Build history of the part. All positions in model axes, mm. Round coordinates to 2 decimals unless told otherwise and drop trailing zeros. Order: outer loops, then holes, each group sorted by start corner. A loop starts at its lowest first (then second) coordinate and runs counter-clockwise, first axis right, second up. Notation, with made-up numbers: (-15.5, 61.5) - (-9.5, 61.5) arc R24 ccw to (-9.5, 98.5) - close; hole circle Ø5 at (-25.75, -29.5). An arc over 180 degrees is marked (long way). Write each question's results on one line, items separated by ' | '. Start each with the question number.
```python
from build123d import *

# Parameters (mm, degrees)
SKETCH1_W           = 10.16
SKETCH1_H           = 3.175
BOSS_EXTRUDE1_DEPTH = 3.175


with BuildPart() as part:
    # Sketch1 → Boss-Extrude1 (new body)
    with BuildSketch(Plane(origin=(0, 0, 0), x_dir=(1, 0, 0), z_dir=(0, 1, 0))):
        with Locations((22.86, -42.8625)):
            Rectangle(SKETCH1_W, SKETCH1_H)
        Polygon((27.94, -41.275), (38.1, -41.275), (48.26, -41.275), (58.42, -41.275), (68.58, -41.275), (76.2, -41.275), (76.2, 41.275), (68.58, 41.275), (58.42, 41.275), (48.26, 41.275), (38.1, 41.275), (27.94, 41.275), (17.78, 41.275), (-76.2, 41.275), (-76.2, -41.275), (17.78, -41.275), align=None)
        with Locations((43.18, -42.8625)):
            Rectangle(SKETCH1_W, SKETCH1_H)
        with Locations((22.86, 42.8625)):
            Rectangle(SKETCH1_W, SKETCH1_H)
        with Locations((63.5, -42.8625)):
            Rectangle(SKETCH1_W, SKETCH1_H)
        with Locations((63.5, 42.8625)):
            Rectangle(SKETCH1_W, SKETCH1_H)
        with Locations((43.18, 42.8625)):
            Rectangle(SKETCH1_W, SKETCH1_H)
    extrude(amount=BOSS_EXTRUDE1_DEPTH)


solid = part.part
```
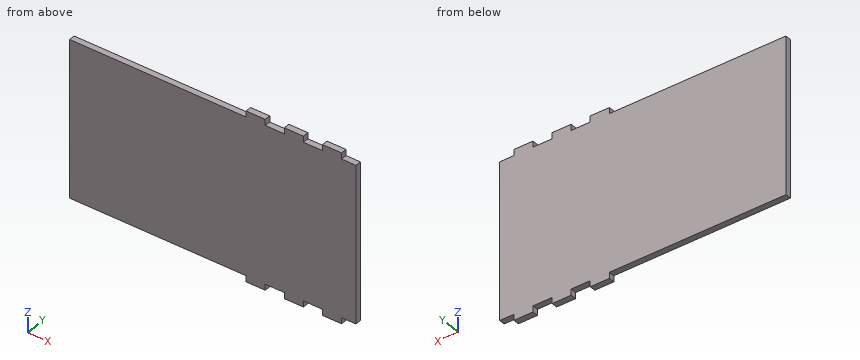
1. Wall check: line 1 (Z direction, x = 6, y = 0.95) (3 decimals). Give the ranges that are in metal, low to high. Write a range as from..to.
2. Cut at A-A (y = 1.45). List the corners of the cut face in (x, z) (3 decimals), plus the area to 3 significant figures.
3. Flat gauge pins, fed straight in: pin 1 Ø1 at (y, z) = (1.5, -42.5) entering from -X; pin 2 Ø1.6 at (x, y) = (-34.5, 2) entering from +Z (3 decimals); pin 3 Ø1.6 at (x, y) = (35, 2) entering from -Z (3 decimals). Where does each tip first touch, or does it go through?
4. Cut at B-B (x = 14). List the corners of the cut face in (y, z) (3 decimals).
A:
1) line 1: z = -41.275..41.275
2) outline: (-76.2, -41.275) - (17.78, -41.275) - (17.78, -44.45) - (27.94, -44.45) - (27.94, -41.275) - (38.1, -41.275) - (38.1, -44.45) - (48.26, -44.45) - (48.26, -41.275) - (58.42, -41.275) - (58.42, -44.45) - (68.58, -44.45) - (68.58, -41.275) - (76.2, -41.275) - (76.2, 41.275) - (68.58, 41.275) - (68.58, 44.45) - (58.42, 44.45) - (58.42, 41.275) - (48.26, 41.275) - (48.26, 44.45) - (38.1, 44.45) - (38.1, 41.275) - (27.94, 41.275) - (27.94, 44.45) - (17.78, 44.45) - (17.78, 41.275) - (-76.2, 41.275) - close | area: 12,800 mm^2
3) pin 1: stops at x = 17.78 | pin 2: stops at z = 41.275 | pin 3: stops at z = -41.275
4) outline: (0, -41.275) - (3.175, -41.275) - (3.175, 41.275) - (0, 41.275) - close
